```python
from build123d import *

# Parameters (mm, degrees)
F0_W     = 44
F0_H     = 44
F0_R     = 6.222357
F0_R_2   = 2.778255
F1_DEPTH = 25


with BuildPart() as f1:
    # F0 (on Front) → F1 (new body)
    with BuildSketch(Plane.XZ):
        with Locations((58.216352, 46.031879)):
            Rectangle(F0_W, F0_H)
        with Locations((58.216352, 46.031879)):
            Circle(F0_R, mode=Mode.SUBTRACT)
        with Locations((75.216352, 29.031879)):
            Circle(F0_R_2, mode=Mode.SUBTRACT)
        with Locations((41.216352, 63.031879)):
            Circle(F0_R_2, mode=Mode.SUBTRACT)
    extrude(amount=F1_DEPTH)


solid = f1.part
```
Geometry check sheet. Reference: the model listing, model coordinates, mm. Coordinates: 2 decimals unless noted, no trailing zeros. Order: outer loops, then holes, each group sorted by start corner. A loop starts at its lowest first (then second) coordinate and runs counter-clockwise, first axis right, second up.
Item 1: Mould release check, pull along X, two halves, no side actions. Record for faces 1 (the flat face through (58, -12, 24.032)), 2 (the cylindrical face through (42.71, -12.325, 65.375)), 3 (the flat face through (36.216, -12, 46)): released by +X, released by -X, zero draft, split by the parting line, or undercut.
Item 2: Section check B-B (z = 42.5). Enter the section's corners in (x, y).
Item 3: Section check C-C (y = -15.75). Enter the section's corners in (x, z).
Item 4: Scan lines: line 1 along X through (y, z) = (-11.25, 51); line 2 along Z through (x, y) = (53, -21); line 3 along X through (y, z) = (-3.75, 47.5). Record each from-to range of solid material in increasing order.
Item 5: Section check A-A (x = 39). Enter the section's corners in (y, z), plus the area to 3 significant figures.
Check sheet entries:
1. face 1: zero draft
1. face 2: undercut
1. face 3: released by -X
2. outline: (36.22, -25) - (53.09, -25) - (53.09, 0) - (36.22, 0) - close; (63.34, -25) - (80.22, -25) - (80.22, 0) - (63.34, 0) - close
3. outline: (36.22, 24.03) - (80.22, 24.03) - (80.22, 68.03) - (36.22, 68.03) - close; hole circle Ø5.56 at (41.22, 63.03); hole circle Ø12.44 at (58.22, 46.03); hole circle Ø5.56 at (75.22, 29.03)
4. line 1: x = 36.22 to 54.47, 61.96 to 80.22
4. line 2: z = 24.03 to 42.64, 49.42 to 68.03
4. line 3: x = 36.22 to 52.17, 64.26 to 80.22
5. outline: (-25, 24.03) - (0, 24.03) - (0, 61.36) - (-25, 61.36) - close; (-25, 64.71) - (0, 64.71) - (0, 68.03) - (-25, 68.03) - close
5. area: 1,020 mm2
